```python
from build123d import *

# Parameters (mm, degrees)
SKETCH1_W           = 61
SKETCH1_H           = 41
BOSS_EXTRUDE1_DEPTH = 23
SHELL1_T            = 3
SKETCH2_W           = 67
SKETCH2_H           = 47
CUT_EXTRUDE1_DEPTH  = 23
SKETCH3_W           = 60.7
SKETCH3_H           = 40.7
SKETCH3_W_2         = 57.7
SKETCH3_H_2         = 38.7
BOSS_EXTRUDE2_DEPTH = 11.5
BOSS_EXTRUDE3_START = -10
SKETCH4_R           = 1
BOSS_EXTRUDE3_DEPTH = 20.7
BOSS_EXTRUDE4_START = -10
BOSS_EXTRUDE4_DEPTH = 40.7
FILLET1_R           = 3
FILLET2_R           = 1
FILLET3_SIZE        = 3
FILLET3_SIZE_2      = 0.8


with BuildPart() as part:
    # Sketch1 → Boss-Extrude1 (new body)
    with BuildSketch(Plane(origin=(0, 0, 0), x_dir=(1, 0, 0), z_dir=(0, 1, 0))):
        Rectangle(SKETCH1_W, SKETCH1_H)
    extrude(amount=BOSS_EXTRUDE1_DEPTH)

    # Shell1
    shell1_openings = [part.faces().sort_by_distance(p)[0] for p in [
        (0, 23, 0),
    ]]
    offset(amount=SHELL1_T, openings=shell1_openings, kind=Kind.INTERSECTION)

    # Sketch2 → Cut-Extrude1 (cut)
    with BuildSketch(Plane(origin=(0, 23, 0), x_dir=(1, 0, 0), z_dir=(0, 1, 0))):
        Rectangle(SKETCH2_W, SKETCH2_H)
    extrude(amount=-CUT_EXTRUDE1_DEPTH, mode=Mode.SUBTRACT)

    # Sketch3 → Boss-Extrude2 (add)
    with BuildSketch(Plane(origin=(0, 0, 0), x_dir=(1, 0, 0), z_dir=(0, 1, 0))):
        Rectangle(SKETCH3_W, SKETCH3_H)
        Rectangle(SKETCH3_W_2, SKETCH3_H_2, mode=Mode.SUBTRACT)
    extrude(amount=BOSS_EXTRUDE2_DEPTH)

    # Sketch4 → Boss-Extrude3 (add)
    with BuildSketch(Plane.XY.offset(20.35).offset(BOSS_EXTRUDE3_START)):
        with Locations((-29.85, 6.5)):
            Circle(SKETCH4_R)
        with Locations((29.85, 6.5)):
            Circle(SKETCH4_R)
    extrude(amount=-BOSS_EXTRUDE3_DEPTH)

    # Sketch5 → Boss-Extrude4 (add)
    with BuildSketch(Plane(origin=(30.35, 0, 0), x_dir=(0, 0, -1), z_dir=(1, 0, 0)).offset(BOSS_EXTRUDE4_START)):
        with BuildLine():
            Line((-20.35, 5.633974596), (-20.35, 7.366025404))
            ThreePointArc((-20.35, 7.366025404), (-20.85, 6.5), (-20.35, 5.633974596))
        make_face()
        with BuildLine():
            ThreePointArc((20.35, 5.633974596), (20.716025404, 6), (20.85, 6.5))
            ThreePointArc((20.85, 6.5), (20.716025404, 7), (20.35, 7.366025404))
            Line((20.35, 7.366025404), (20.35, 5.633974596))
        make_face()
    extrude(amount=-BOSS_EXTRUDE4_DEPTH)

    # Fillet1
    fillet1_edges = [part.edges().sort_by_distance(p)[0] for p in [
        (33.5, -1.5, 23.5),
        (-33.5, -1.5, 23.5),
        (-33.5, -1.5, -23.5),
        (33.5, -1.5, -23.5),
    ]]
    fillet(fillet1_edges, radius=FILLET1_R)

    # Fillet2
    fillet2_edges = [part.edges().sort_by_distance(p)[0] for p in [
        (30.35, 5.75, 20.35),
        (30.35, 5.75, -20.35),
        (-30.35, 5.75, -20.35),
        (-30.35, 5.75, 20.35),
    ]]
    fillet(fillet2_edges, radius=FILLET2_R)

    # Fillet3
    # an asymmetric fillet: 3, 0.8 mm, written as the material it takes off along each edge
    with BuildSketch(Plane(origin=(30.35, 11.5, -19.35), x_dir=(0, -1, 0), z_dir=(0, 0, 1)), Plane(origin=(-30.35, 11.5, 19.35), x_dir=(0, -1, 0), z_dir=(0, 0, -1))) as fillet3_piece_1:
        with BuildLine():
            Bezier((FILLET3_SIZE, 0), (0, 0), (0, -FILLET3_SIZE_2), weights=[1, 0.707106781, 1])
            Line((0, -FILLET3_SIZE_2), (0, 0))
            Line((0, 0), (FILLET3_SIZE, 0))
        make_face()
    extrude(amount=38.7, mode=Mode.SUBTRACT)
    with BuildSketch(Plane(origin=(29.35, 11.5, -19.35), x_dir=(0, 0, -1), z_dir=(-1, 0, 0))) as fillet3_piece_2:
        with BuildLine():
            Bezier((1, FILLET3_SIZE), (1, 0), (1 - FILLET3_SIZE_2, 0), weights=[1, 0.707106781, 1])
            Line((1 - FILLET3_SIZE_2, 0), (1, 0))
            Line((1, 0), (1, FILLET3_SIZE))
        make_face()
    revolve(axis=Axis((29.35, 11.5, -19.35), (0, -1, 0)), revolution_arc=90, mode=Mode.SUBTRACT)
    with BuildSketch(Plane(origin=(29.35, 11.5, 19.35), x_dir=(1, 0, 0), z_dir=(0, 0, -1))) as fillet3_piece_3:
        with BuildLine():
            Bezier((1, FILLET3_SIZE), (1, 0), (1 - FILLET3_SIZE_2, 0), weights=[1, 0.707106781, 1])
            Line((1 - FILLET3_SIZE_2, 0), (1, 0))
            Line((1, 0), (1, FILLET3_SIZE))
        make_face()
    revolve(axis=Axis((29.35, 11.5, 19.35), (0, -1, 0)), revolution_arc=90, mode=Mode.SUBTRACT)
    with BuildSketch(Plane(origin=(-29.35, 11.5, -20.35), x_dir=(0, -1, 0), z_dir=(1, 0, 0)), Plane(origin=(29.35, 11.5, 20.35), x_dir=(0, -1, 0), z_dir=(-1, 0, 0))) as fillet3_piece_4:
        with BuildLine():
            Bezier((FILLET3_SIZE, 0), (0, 0), (0, -FILLET3_SIZE_2), weights=[1, 0.707106781, 1])
            Line((0, -FILLET3_SIZE_2), (0, 0))
            Line((0, 0), (FILLET3_SIZE, 0))
        make_face()
    extrude(amount=58.7, mode=Mode.SUBTRACT)
    with BuildSketch(Plane(origin=(-29.35, 11.5, -19.35), x_dir=(0, 0, -1), z_dir=(1, 0, 0))) as fillet3_piece_5:
        with BuildLine():
            Bezier((1, -FILLET3_SIZE), (1, 0), (1 - FILLET3_SIZE_2, 0), weights=[1, 0.707106781, 1])
            Line((1 - FILLET3_SIZE_2, 0), (1, 0))
            Line((1, 0), (1, -FILLET3_SIZE))
        make_face()
    revolve(axis=Axis((-29.35, 11.5, -19.35), (0, 1, 0)), revolution_arc=90, mode=Mode.SUBTRACT)
    with BuildSketch(Plane(origin=(-29.35, 11.5, 19.35), x_dir=(0, 0, 1), z_dir=(1, 0, 0))) as fillet3_piece_6:
        with BuildLine():
            Bezier((1, FILLET3_SIZE), (1, 0), (1 - FILLET3_SIZE_2, 0), weights=[1, 0.707106781, 1])
            Line((1 - FILLET3_SIZE_2, 0), (1, 0))
            Line((1, 0), (1, FILLET3_SIZE))
        make_face()
    revolve(axis=Axis((-29.35, 11.5, 19.35), (0, -1, 0)), revolution_arc=90, mode=Mode.SUBTRACT)


solid = part.part
```
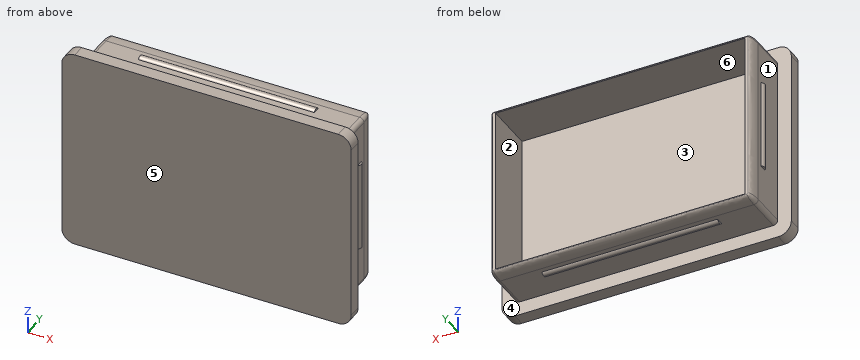
Input: part model. Units: mm. Frame: model coordinates. Face numbers are marked on the shaded views. A direction names the side the tool comes from. Give positions to 0.01 mm unless a question says otherwise; leave off trailing zeros. Order: outer loops, then holes, each group sorted by start corner. A loop starts at its lowest first (then second) coordinate and runs counter-clockwise, first axis right, second up. Notation, with made-up numbers: (19.5, -20) -> (65.5, -20) arc R17 cw to (65.5, -7) -> close; hole circle Ø11 at (55, -19.75). An arc over 180 degrees is marked (long way). Write each question's results on one line, items separated by ' | '. Start each with the question number.
Item 1: Line query: line 1 (X direction, y = 7.5, z = 10.5); line 2 (Z direction, x = -14, y = 3.75). Output: solid intervals per line, ascending.
Item 2: Contact query for flat-ended pins moving along their axis: P1, Ø4, axis at x = 10, y = 6, coming from the +Z side; P2, Ø6, axis at y = 5.5, z = 10, coming from the +X side; P3, Ø3.5, axis at y = 4.5, z = 5.5, coming from the +X side. Output: stop coordinate, or through.
Item 3: Set-up query: the marked faces 4, 5 and 6. Return all of +Z, -Z, +X, -X, +Y, -Y with unobstructed straight access to the full face (end or side cutting, diameter ignored); none if empty.
Item 4: Mould query, pull axis Y, two halves, no side actions, for the marked faces 1, 2 and 3. Classes: pulls with the +Y half, pulls with the -Y half, needs draft (parallel to the pull), parting line crosses it, or undercut.
Item 5: Cut plane A-A on y = 4. Return the cut outline in (x, z).
Established:
1) line 1: -30.35 to -28.85, 28.85 to 30.35 | line 2: -20.35 to -19.35, 19.35 to 20.35
2) P1: z = 20.85 | P2: x = 30.85 | P3: x = 30.82
3) face 4: none | face 5: +Z, -Z, +X, -X, -Y | face 6: +Y
4) face 1: undercut | face 2: needs draft | face 3: pulls with the +Y half
5) outline: (-30.35, -19.35) arc R1 ccw to (-29.35, -20.35) -> (29.35, -20.35) arc R1 ccw to (30.35, -19.35) -> (30.35, 19.35) arc R1 ccw to (29.35, 20.35) -> (-29.35, 20.35) arc R1 ccw to (-30.35, 19.35) -> close; hole (-28.85, -19.35) -> (28.85, -19.35) -> (28.85, 19.35) -> (-28.85, 19.35) -> close
